```python
from build123d import *

# Parameters (mm, degrees)
CROQUIS1_W              = 283.41300437
CROQUIS1_H              = 39.51255033
CROQUIS1_R              = 10
SALIENTE_EXTRUIR1_DEPTH = 10


with BuildPart() as part:
    # Croquis1 → Saliente-Extruir1 (new body)
    with BuildSketch(Plane.XY):
        Rectangle(CROQUIS1_W, CROQUIS1_H)
        Circle(CROQUIS1_R, mode=Mode.SUBTRACT)
        with Locations((120, 0)):
            Circle(CROQUIS1_R, mode=Mode.SUBTRACT)
    extrude(amount=SALIENTE_EXTRUIR1_DEPTH)


solid = part.part
```
Can you work these out from the model? Positions are in its coordinate system, mm. Coordinates: 2 decimals unless noted, no trailing zeros. Loops run counter-clockwise (first coordinate to the right, second up) from the corner with the lowest first, then second, coordinate; pieces in that order, holes last. Notation, with made-up numbers: M -17.75,44 L 39.25,44 A9 cw 39.25,60 Z; hole C -35.5,71.5 d9. An arc over 180 degrees is marked long. Put each result on its own line as item: value. Start each with the question number.
(1) Will this pin go through, and if not, where does the flat tip stop? pin 1 Ø12 at (x, y) = (85.5, 1) entering from -Z.
(2) Imagine slicing it at A-A on x = 120. List the corners of the cut face in (y, z) for me.
(3) I need wall thicknesses on probe 1 along Y at (x, z) = (120, 3); probe 2 along X at (y, z) = (-3.5, 1.25); probe 3 along X at (y, z) = (-7, 8.5). Which ranges of each line are inside material? Lowest first, please.
(4) We'd pull the mould along Y, two halves only. Please class faces 1 (the face through (110, 0, 5)), 2 (the face through (-2, -13, 0)), 3 (the face through (-2, -19.756, 5)): +Y half, -Y half, draft (parallel to the pull), parting line (faces both ways), or undercut.
(5) Imagine slicing it at C-C on z = 3.25. List the corners of the cut face in (x, y) for me, and give its area (3 significant figures).
(6) Imagine slicing it at B-B on y = 0. List the corners of the cut face in (x, z) for me.
Worked answers:
1. pin 1: stops at z = 0
2. outline: M -19.76,0 L -10,0 L -10,10 L -19.76,10 Z; M 10,0 L 19.76,0 L 19.76,10 L 10,10 Z
3. probe 1: y = -19.76 to -10, 10 to 19.76
3. probe 2: x = -141.71 to -9.37, 9.37 to 110.63, 129.37 to 141.71
3. probe 3: x = -141.71 to -7.14, 7.14 to 112.86, 127.14 to 141.71
4. face 1: undercut
4. face 2: draft
4. face 3: -Y half
5. outline: M -141.71,-19.76 L 141.71,-19.76 L 141.71,19.76 L -141.71,19.76 Z; hole C 0,0 d20; hole C 120,0 d20
5. area: 10,600 mm2
6. outline: M -141.71,0 L -10,0 L -10,10 L -141.71,10 Z; M 10,0 L 110,0 L 110,10 L 10,10 Z; M 130,0 L 141.71,0 L 141.71,10 L 130,10 Z
